```python
from build123d import *

# Parameters (mm, degrees)
EXTRUDE_1_DEPTH          = 120
SKETCH_2_R               = 1.6
CUT_EXTRUDE_1_DEPTH      = 120
SKETCH_3_R               = 1.6
CUT_EXTRUDE_2_DEPTH      = 10
SKETCH_4_R               = 1.1
CUT_EXTRUDE_3_DEPTH      = 12
SKETCH_5_W               = 11
SKETCH_5_H               = 120
EXTRUDE_2_DEPTH          = 2
SKETCH_6_W               = 49
SKETCH_6_H               = 30
CUT_EXTRUDE_4_DEPTH      = 10
CUT_EXTRUDE_5_DEPTH      = 42
CUT_EXTRUDE_5_DEPTH_BACK = 16
SKETCH_7_W               = 3
SKETCH_7_H               = 30
CUT_EXTRUDE_6_DEPTH      = 35
CUT_EXTRUDE_6_DEPTH_BACK = 11
SKETCH_8_W               = 52
SKETCH_8_H               = 12
SKETCH_9_W               = 2
SKETCH_9_H               = 42
CUT_EXTRUDE_7_DEPTH      = 20
SKETCH_10_W              = 11
SKETCH_10_H              = 54
CUT_EXTRUDE_8_DEPTH      = 10
SKETCH_11_W              = 11
SKETCH_11_H              = 68
SKETCH_11_R              = 1.6
EXTRUDE_3_DEPTH          = 1
SKETCH_12_W              = 11
SKETCH_12_H              = 1
CUT_EXTRUDE_9_DEPTH      = 91
CUT_EXTRUDE_10_DEPTH     = 10
SKETCH_14_W              = 35
SKETCH_14_H              = 6
CUT_EXTRUDE_11_DEPTH     = 10
FILLET_1_R               = 2
FILLET_2_R               = 1


with BuildPart() as part:
    # 草图1 → 凸台-拉伸1 (new body)
    with BuildSketch(Plane(origin=(0, 0, 0), x_dir=(1, 0, 0), z_dir=(0, 1, 0))):
        Polygon((0, 0), (8, 0), (8, -3), (-3, -3), (-3, 49), (0, 49), align=None)
    extrude(amount=EXTRUDE_1_DEPTH)

    # 草图2 → 切除-拉伸1 (cut)
    with BuildSketch(Plane(origin=(0, 0, 0), x_dir=(-1, 0, 0), z_dir=(0, 0, -1))):
        with Locations((-4.5, 60)):
            Circle(SKETCH_2_R)
        with Locations((-4.5, 45)):
            Circle(SKETCH_2_R)
        with Locations((-4.5, 30)):
            Circle(SKETCH_2_R)
        with Locations((-4.5, 15)):
            Circle(SKETCH_2_R)
        with Locations((-4.5, 75)):
            Circle(SKETCH_2_R)
        with Locations((-4.5, 90)):
            Circle(SKETCH_2_R)
        with Locations((-4.5, 105)):
            Circle(SKETCH_2_R)
    cut_extrude_1 = extrude(amount=-CUT_EXTRUDE_1_DEPTH, mode=Mode.SUBTRACT)

    # 草图3 → 切除-拉伸2 (cut)
    with BuildSketch(Plane(origin=(0, 0, 0), x_dir=(0, 0, -1), z_dir=(1, 0, 0))):
        with Locations((14.5, 7.384470662)):
            Circle(SKETCH_3_R)
        with Locations((14.5, 22.384470662)):
            Circle(SKETCH_3_R)
        with Locations((14.5, 37.384470662)):
            Circle(SKETCH_3_R)
        with Locations((14.5, 52.384470662)):
            Circle(SKETCH_3_R)
        with Locations((14.5, 67.384470662)):
            Circle(SKETCH_3_R)
        with Locations((34.5, 67.384470662)):
            Circle(SKETCH_3_R)
        with Locations((34.5, 52.384470662)):
            Circle(SKETCH_3_R)
        with Locations((34.5, 37.384470662)):
            Circle(SKETCH_3_R)
        with Locations((34.5, 22.384470662)):
            Circle(SKETCH_3_R)
        with Locations((34.5, 7.384470662)):
            Circle(SKETCH_3_R)
    extrude(amount=-CUT_EXTRUDE_2_DEPTH, mode=Mode.SUBTRACT)

    # 草图4 → 切除-拉伸3 (cut)
    with BuildSketch(Plane(origin=(0, 0, 0), x_dir=(0, 0, -1), z_dir=(1, 0, 0))):
        with Locations((15.7, 117)):
            Circle(SKETCH_4_R)
        with Locations((33.3, 117)):
            Circle(SKETCH_4_R)
        with Locations((24.5, 79.8)):
            Circle(SKETCH_4_R)
    extrude(amount=-CUT_EXTRUDE_3_DEPTH, mode=Mode.SUBTRACT)

    # 草图5 → 凸台-拉伸2 (add)
    with BuildSketch(Plane(origin=(0, 0, -49), x_dir=(-1, 0, 0), z_dir=(0, 0, -1))):
        with Locations((-2.5, 60)):
            Rectangle(SKETCH_5_W, SKETCH_5_H)
    extrude(amount=EXTRUDE_2_DEPTH)

    # 镜向3: 切除-拉伸1 across plane
    add(cut_extrude_1.mirror(Plane(origin=(0, 0, -24.5), x_dir=(1, 0, 0), z_dir=(0, 0, -1))), mode=Mode.SUBTRACT)

    # 草图6 → 切除-拉伸4 (cut)
    with BuildSketch(Plane(origin=(0, 0, 0), x_dir=(0, 0, -1), z_dir=(1, 0, 0))):
        with Locations((24.5, 15)):
            Rectangle(SKETCH_6_W, SKETCH_6_H)
    extrude(amount=-CUT_EXTRUDE_4_DEPTH, mode=Mode.SUBTRACT)

    # 草图7 → 切除-拉伸5 (cut, two sides: drawn at the far end of the back side and taken through both)
    with BuildSketch(Plane(origin=(0, 0, 0), x_dir=(0, 0, -1), z_dir=(1, 0, 0)).offset(-CUT_EXTRUDE_5_DEPTH_BACK)):
        with Locations((-1.5, 15)):
            Rectangle(SKETCH_7_W, SKETCH_7_H)
    extrude(amount=CUT_EXTRUDE_5_DEPTH + CUT_EXTRUDE_5_DEPTH_BACK, mode=Mode.SUBTRACT)

    # 草图8 → 切除-拉伸6 (cut, two sides: drawn at the far end of the back side and taken through both)
    with BuildSketch(Plane(origin=(0, 0, 0), x_dir=(0, 0, -1), z_dir=(1, 0, 0)).offset(-CUT_EXTRUDE_6_DEPTH_BACK)):
        with Locations((23, 36)):
            Rectangle(SKETCH_8_W, SKETCH_8_H)
    extrude(amount=CUT_EXTRUDE_6_DEPTH + CUT_EXTRUDE_6_DEPTH_BACK, mode=Mode.SUBTRACT)

    # 草图9 → 切除-拉伸7 (cut)
    with BuildSketch(Plane.ZY.offset(3)):
        with Locations((-50, 21)):
            Rectangle(SKETCH_9_W, SKETCH_9_H)
    extrude(amount=-CUT_EXTRUDE_7_DEPTH, mode=Mode.SUBTRACT)

    # 草图10 → 切除-拉伸8 (cut)
    with BuildSketch(Plane(origin=(0, 120, 0), x_dir=(1, 0, 0), z_dir=(0, 1, 0))):
        with Locations((2.5, 24)):
            Rectangle(SKETCH_10_W, SKETCH_10_H)
    extrude(amount=-CUT_EXTRUDE_8_DEPTH, mode=Mode.SUBTRACT)

    # 草图11 → 凸台-拉伸3 (add)
    with BuildSketch(Plane(origin=(0, 0, -51), x_dir=(-1, 0, 0), z_dir=(0, 0, -1))):
        with Locations((-2.5, 76)):
            Rectangle(SKETCH_11_W, SKETCH_11_H)
        with Locations((-4.5, 105)):
            Circle(SKETCH_11_R, mode=Mode.SUBTRACT)
        with Locations((-4.5, 45)):
            Circle(SKETCH_11_R, mode=Mode.SUBTRACT)
        with Locations((-4.5, 60)):
            Circle(SKETCH_11_R, mode=Mode.SUBTRACT)
        with Locations((-4.5, 75)):
            Circle(SKETCH_11_R, mode=Mode.SUBTRACT)
        with Locations((-4.5, 90)):
            Circle(SKETCH_11_R, mode=Mode.SUBTRACT)
    extrude(amount=EXTRUDE_3_DEPTH)

    # 草图12 → 切除-拉伸9 (cut)
    with BuildSketch(Plane(origin=(0, 110, 0), x_dir=(1, 0, 0), z_dir=(0, 1, 0))):
        with Locations((2.5, -2.5)):
            Rectangle(SKETCH_12_W, SKETCH_12_H)
    extrude(amount=-CUT_EXTRUDE_9_DEPTH, mode=Mode.SUBTRACT)

    # 草图13 → 切除-拉伸10 (cut)
    with BuildSketch(Plane.ZY.offset(3)):
        Polygon((-31.5, 66.326548237), (-24.5, 75.017418774), (-17.5, 66.326548237), (-17.5, 55.384470662), (-31.5, 55.384470662), align=None)
    extrude(amount=-CUT_EXTRUDE_10_DEPTH, mode=Mode.SUBTRACT)

    # 草图14 → 切除-拉伸11 (cut)
    with BuildSketch(Plane.ZY.offset(3)):
        with Locations((-24.5, 97.5)):
            Rectangle(SKETCH_14_W, SKETCH_14_H)
        with BuildLine():
            Line((-22.018065271, 79.5), (-7, 79.5))
            Line((-7, 79.5), (-7, 85.5))
            Line((-7, 85.5), (-42, 85.5))
            Line((-42, 85.5), (-42, 79.5))
            Line((-42, 79.5), (-26.981934729, 79.5))
            ThreePointArc((-26.981934729, 79.5), (-24.5, 82.3), (-22.018065271, 79.5))
        make_face()
    extrude(amount=-CUT_EXTRUDE_11_DEPTH, mode=Mode.SUBTRACT)

    # 圆角1
    fillet_1_edges = [part.edges().sort_by_distance(p)[0] for p in [
        (-1.5, 55.384470662, -31.5),
        (-1.5, 66.326548237, -31.5),
        (-1.5, 75.017418774, -24.5),
        (-1.5, 66.326548237, -17.5),
        (-1.5, 55.384470662, -17.5),
        (-1.5, 100.5, -7),
        (-1.5, 94.5, -7),
        (-1.5, 94.5, -42),
        (-1.5, 100.5, -42),
        (-1.5, 85.5, -7),
        (-1.5, 79.5, -7),
        (-1.5, 79.5, -22.018065271),
        (-1.5, 79.5, -26.981934729),
        (-1.5, 79.5, -42),
        (-1.5, 85.5, -42),
    ]]
    fillet(fillet_1_edges, radius=FILLET_1_R)

    # 圆角2
    fillet_2_edges = [part.edges().sort_by_distance(p)[0] for p in [
        (0, 76, -49),
        (0, 76, 0),
    ]]
    fillet(fillet_2_edges, radius=FILLET_2_R)


solid = part.part
```
Design review of the part built by this model. Coordinates are the model's own, in mm. A direction names the side the tool comes from. Coordinates: 2 decimals unless noted, no trailing zeros. Write each loop counter-clockwise with the first axis right and the second up, starting at its lowest first coordinate (ties: lowest second). Pieces come first, ordered by that corner, then holes.
1) Insertion check: pin 1 (2 mm diameter, centred on x = 5, y = 61, fed in from -Z); pin 2 (8 mm diameter, centred on y = 102, z = -41, fed in from +X). Each pin has a flat end and moves straight along its axis. Give the tip position at first contact, or say it passes through.
2) Add section A-A (z = -14.5). Write out the cut boundary in (x, y).
3) Mouldability with a two-part tool opening along X and no side actions: class faces 1 (the cylindrical face through (-1.48, 80.07, -41.4)), 2 (the flat face through (8, 76, 1)), 3 (the cylindrical face through (4.708, 76.586, 0.986)) as +X half, -X half, draft (parallel to the pull), parting line (faces both ways), or undercut.
4) To check wall thickness, follow L1, parallel to Y at x = -2.25, z = -14.5; L2, parallel to Z at x = 4.75, y = 95; L3, parallel to X at y = 90, z = -50.9. State the ranges of each line that lie inside material, in increasing order.
5) Machinability: for faces 4 (the cylindrical face through (-1.48, 84.93, -7.6)), 5 (the cylindrical face through (4.708, 91.586, -50.479)), which of the approach directions +Z, -Z, +X, -X, +Y, -Y give a long, thin tool a straight path to every point of the face, cutting with its end or side? Answer none if there is none.
6) Add section B-B (y = 60). Write out the cut boundary in (x, z).
7) Add section C-C (y = 90). Write out the cut boundary in (x, z), plus the area to 3 significant figures.
8) Add section D-D (y = 99.5). Write out the cut boundary in (x, z).
Check result:
1. pin 1: stops at z = -52
1. pin 2: stops at x = 0
2. outline: (-3, 42) - (0, 42) - (0, 50.78) - (-3, 50.78) - close; (-3, 53.98) - (0, 53.98) - (0, 65.78) - (-3, 65.78) - close; (-3, 68.98) - (0, 68.98) - (0, 79.5) - (-3, 79.5) - close; (-3, 85.5) - (0, 85.5) - (0, 94.5) - (-3, 94.5) - close; (-3, 100.5) - (0, 100.5) - (0, 110) - (-3, 110) - close
3. face 1: draft
3. face 2: +X half
3. face 3: undercut
4. L1: y = 42 to 50.78, 53.98 to 65.78, 68.98 to 79.5, 85.5 to 94.5, 100.5 to 110
4. L2: z = -52 to -49, 0 to 2
4. L3: x = -3 to 2.9, 6.1 to 8
5. face 4: +X, -X
5. face 5: +Z, -Z
6. outline: (-3, -52) - (2.9, -52) - (2.9, -49) - (1, -49) arc R1 cw to (0, -48) - (0, -31.5) - (-3, -31.5) - close; (-3, -17.5) - (0, -17.5) - (0, -1) arc R1 cw to (1, 0) - (2.9, 0) - (2.9, 2) - (-3, 2) - close; (6.1, -52) - (8, -52) - (8, -49) - (6.1, -49) - close; (6.1, 0) - (8, 0) - (8, 2) - (6.1, 2) - close
7. outline: (-3, -52) - (2.9, -52) - (2.9, -49) - (1, -49) arc R1 cw to (0, -48) - (0, -1) arc R1 cw to (1, 0) - (2.9, 0) - (2.9, 2) - (-3, 2) - close; (6.1, -52) - (8, -52) - (8, -49) - (6.1, -49) - close; (6.1, 0) - (8, 0) - (8, 2) - (6.1, 2) - close
7. area: 186 mm2
8. outline: (-3, -52) - (8, -52) - (8, -49) - (1, -49) arc R1 cw to (0, -48) - (0, -41.73) - (-3, -41.73) - close; (-3, -7.27) - (0, -7.27) - (0, -1) arc R1 cw to (1, 0) - (8, 0) - (8, 2) - (-3, 2) - close
